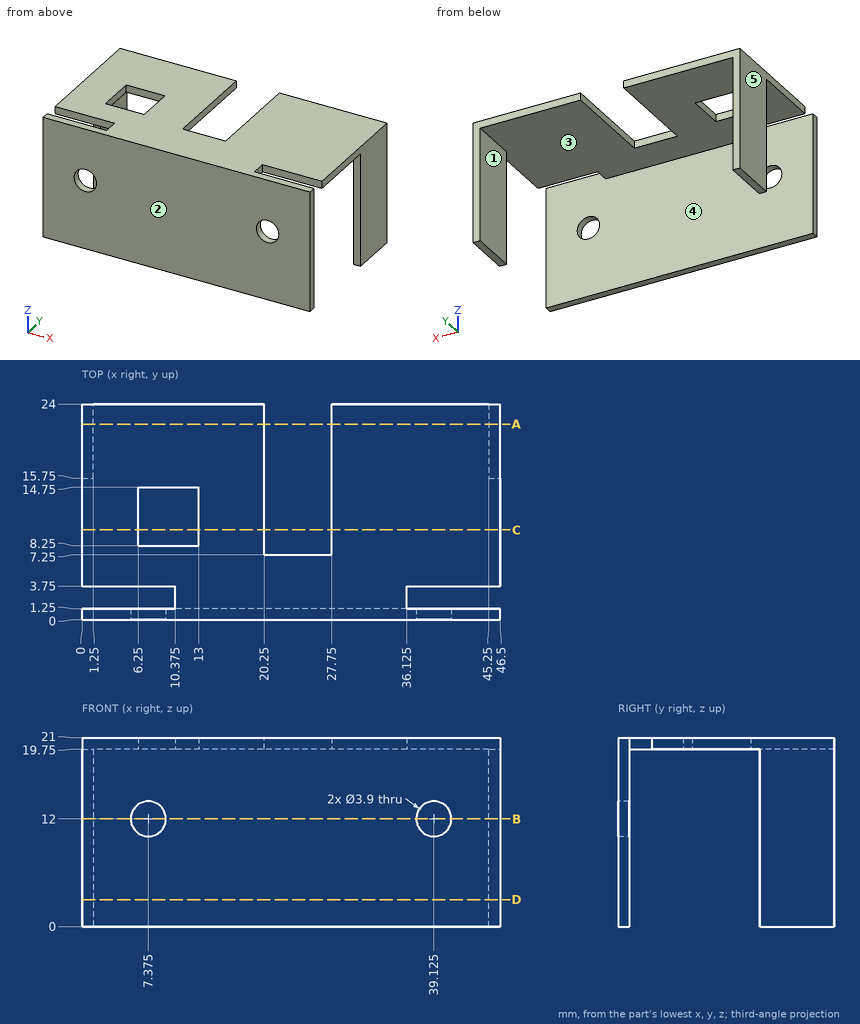
Geometry check sheet. Reference: drawing and pictorial views, mm from the part's lowest x, y, z. A direction names the side the tool comes from. Give positions to 0.01 mm unless a question says otherwise; leave off trailing zeros. Order: outer loops, then holes, each group sorted by start corner. A loop starts at its lowest first (then second) coordinate and runs counter-clockwise, first axis right, second up. Notation, with made-up numbers: M -19.5,2.25 L -3.5,2.25 A34 ccw -3.5,35.25 Z; hole C 64,-34.5 d1. An arc over 180 degrees is marked long. Return JSON: item names as keys, results as strings. Group by question number.
1) Go/stop test with flat-tipped pins: pin 1 Ø3.5 at (x, z) = (7.375, 12) entering from +Y; pin 2 Ø12 at (x, y) = (16, 11) entering from -Z; pin 3 Ø5 at (x, z) = (39.125, 12) entering from +Y; pin 4 Ø1.4 at (y, z) = (2.5, 20.5) entering from -X (3 decimals). Record where each tip stops, or that it passes through.
2) Scan lines: line 1 (X direction, y = 1, z = 12) (3 decimals); line 2 (X direction, y = 12.25, z = 20); line 3 (Z direction, x = 35.5, y = 12.75). Record each from-to range of solid material in increasing order.
3) Section check C-C on y = 10. Record the cut outline in (x, z), and give its area (3 significant figures).
4) Section check B-B on z = 12. Record the cut outline in (x, y) (3 decimals), and give its area (3 significant figures).
5) Mould release check, pull along X, two halves, no side actions. Record for the marked faces 3, 4 and 5: pulls with the +X half, pulls with the -X half, needs draft (parallel to the pull), parting line crosses it, or undercut.
6) Access from +Z, -Z, +X, -X, +Y, -Y to the whole of each face (thin tool, end or side, straight path). Record for the marked faces 1 and 2.
7) Section check D-D on z = 3. Record the cut outline in (x, y), and give its area (4 significant figures).
8) Section check A-A on y = 21.75. Record the cut outline in (x, z).
Answer block:
{
 "1": {"pin 1": "passes through", "pin 2": "stops at z = 19.75", "pin 3": "stops at y = 1.25", "pin 4": "stops at x = 10.375"},
 "2": {"line 1": "x = 0 to 5.425, 9.325 to 37.175, 41.075 to 46.5", "line 2": "x = 0 to 6.25, 13 to 20.25, 27.75 to 46.5", "line 3": "z = 19.75 to 21"},
 "3": {"outline": "M 0,19.75 L 6.25,19.75 L 6.25,21 L 0,21 Z; M 13,19.75 L 20.25,19.75 L 20.25,21 L 13,21 Z; M 27.75,19.75 L 46.5,19.75 L 46.5,21 L 27.75,21 Z", "area": "40.3 mm^2"},
 "4": {"outline": "M 0,0 L 5.425,0 L 5.425,1.25 L 0,1.25 Z; M 0,15.75 L 1.25,15.75 L 1.25,24 L 0,24 Z; M 9.325,0 L 37.175,0 L 37.175,1.25 L 9.325,1.25 Z; M 41.075,0 L 46.5,0 L 46.5,1.25 L 41.075,1.25 Z; M 45.25,15.75 L 46.5,15.75 L 46.5,24 L 45.25,24 Z", "area": "69.0 mm^2"},
 "5": {"face 3": "undercut", "face 4": "needs draft", "face 5": "pulls with the -X half"},
 "6": {"face 1": "-Z, +Y", "face 2": "+Z, -Z, +X, -X, -Y"},
 "7": {"outline": "M 0,0 L 46.5,0 L 46.5,1.25 L 0,1.25 Z; M 0,15.75 L 1.25,15.75 L 1.25,24 L 0,24 Z; M 45.25,15.75 L 46.5,15.75 L 46.5,24 L 45.25,24 Z", "area": "78.75 mm^2"},
 "8": {"outline": "M 0,0 L 1.25,0 L 1.25,19.75 L 20.25,19.75 L 20.25,21 L 0,21 Z; M 27.75,19.75 L 45.25,19.75 L 45.25,0 L 46.5,0 L 46.5,21 L 27.75,21 Z"}
}
